from build123d import *

# Parameters (mm, degrees)
F1_DEPTH = 25
F2_R     = 1
F3_R     = 5


with BuildPart() as f1:
    # F0 (on Front) → F1 (new body)
    with BuildSketch(Plane.XZ):
        with BuildLine():
            Line((129.688292, 40), (-77.611708, 40))
            Line((-77.611708, 40), (-80.730383, 25.327786))
            Line((-80.730383, 25.327786), (-85.744501, 26.39357))
            ThreePointArc((-85.744501, 26.39357), (-100.427997, 26.447621), (-86.991972, 20.524684))
            Line((-86.991972, 20.524684), (-81.977854, 19.4589))
            Line((-81.977854, 19.4589), (-86.11397, 0))
            Line((-86.11397, 0), (138.190554, 0))
            Line((138.190554, 0), (134.054437, 19.4589))
            Line((134.054437, 19.4589), (139.068556, 20.524684))
            ThreePointArc((139.068556, 20.524684), (152.504581, 26.447621), (137.821085, 26.39357))
            Line((137.821085, 26.39357), (132.806967, 25.327786))
            Line((132.806967, 25.327786), (129.688292, 40))
        make_face()
    extrude(amount=F1_DEPTH)

    # F2
    f2_edges = [f1.edges().sort_by_distance(p)[0] for p in [
        (134.054437, -12.5, 19.4589),
        (139.068556, -12.5, 20.524684),
        (132.806967, -12.5, 25.327786),
        (137.821085, -12.5, 26.39357),
        (-85.744501, -12.5, 26.39357),
        (-80.730383, -12.5, 25.327786),
        (-81.977854, -12.5, 19.4589),
        (-86.991972, -12.5, 20.524684),
    ]]
    fillet(f2_edges, radius=F2_R)

    # F3
    f3_edges = [f1.edges().sort_by_distance(p)[0] for p in [
        (26.038292, -25, 0),
        (26.038292, 0, 0),
    ]]
    fillet(f3_edges, radius=F3_R)


solid = f1.part
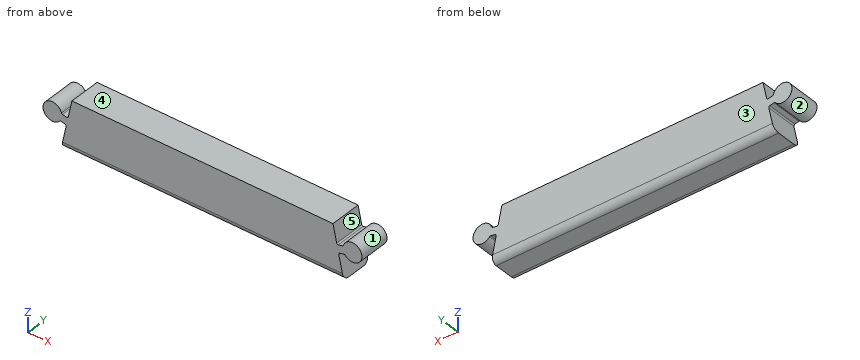
Model file for the job. Use its own axes, mm. Face numbers are marked on the shaded views. A direction names the side the tool comes from. Give positions to 0.01 mm unless a question says otherwise; leave off trailing zeros. Order: outer loops, then holes, each group sorted by start corner. A loop starts at its lowest first (then second) coordinate and runs counter-clockwise, first axis right, second up. Notation, with made-up numbers: M -20,73.25 L -15,73.25 A16 ccw -15,102.25 Z; hole C -37,13.25 d2. An arc over 180 degrees is marked long. Put each result on its own line as item: value. Start each with the question number.
(1) Band-saw the part on C-C on z = 9.5. Give the cut face in (x, y), then the cut area to 3 significant figures.
(2) Tool access for the marked faces 4 and 5: list every direction of +Z, -Z, +X, -X, +Y, -Y with a clear straight run to the whole face (end or side of a thin tool).
(3) Drill centre lines: L1, parallel to X at y = -3, z = 30; L2, parallel to X at y = -18, z = 27; L3, parallel to Z at x = 80, y = -4.5. Where is each one in solid material? Low to high. Write a range as [from, to].
(4) Pull direction X, two halves, no side cores. Call the marked faces 1, 2 and 3: released by +X, released by -X, zero draft, split by the parting line, or undercut.
(5) Band-saw the part on B-B on z = 30. Give the cut face in (x, y), then the cut area to 3 significant figures.
(6) Band-saw the part on A-A on y = -11.5. Give the cut face in (x, z), then the cut area to 3 significant figures.
(7) Pin check, flat tips, straight feed: pin 1 Ø8 at (y, z) = (-6.5, 33.5) entering from +X; pin 2 Ø2 at (y, z) = (-22, 19) entering from -X. Stop position of each tip, or through.
Results below:
1. outline: M -84.09,-25 L 136.17,-25 L 136.17,0 L -84.09,0 Z
1. area: 5,510 mm2
2. face 4: +Z, +X, -X, +Y, -Y
2. face 5: +Z, +Y, -Y
3. L1: x = [-98.58, -87.6], [-79.74, 131.81], [139.68, 150.66]
3. L2: x = [-100.29, -85.9], [-80.37, 132.45], [137.97, 152.37]
3. L3: z = [0.03, 40]
4. face 1: undercut
4. face 2: undercut
4. face 3: zero draft
5. outline: M -98.58,-25 L -87.6,-25 L -87.6,0 L -98.58,0 Z; M -79.74,-25 L 131.81,-25 L 131.81,0 L -79.74,0 Z; M 139.68,-25 L 150.66,-25 L 150.66,0 L 139.68,0 Z
5. area: 5,840 mm2
6. outline: M -87.35,20.06 A1 cw -86.38,20.39 L -82.96,19.67 A1 cw -82.19,18.48 L -86.11,0 L 138.19,0 L 134.26,18.48 A1 cw 135.03,19.67 L 138.46,20.39 A1 cw 139.43,20.06 A7.5 ccw long 137.96,26.96 A1 cw 137.21,26.26 L 133.79,25.54 A1 cw 132.6,26.31 L 129.69,40 L -77.61,40 L -80.52,26.31 A1 cw -81.71,25.54 L -85.13,26.26 A1 cw -85.89,26.96 A7.5 ccw long Z
6. area: 9,040 mm2
7. pin 1: stops at x = 151.08
7. pin 2: stops at x = -98.78
